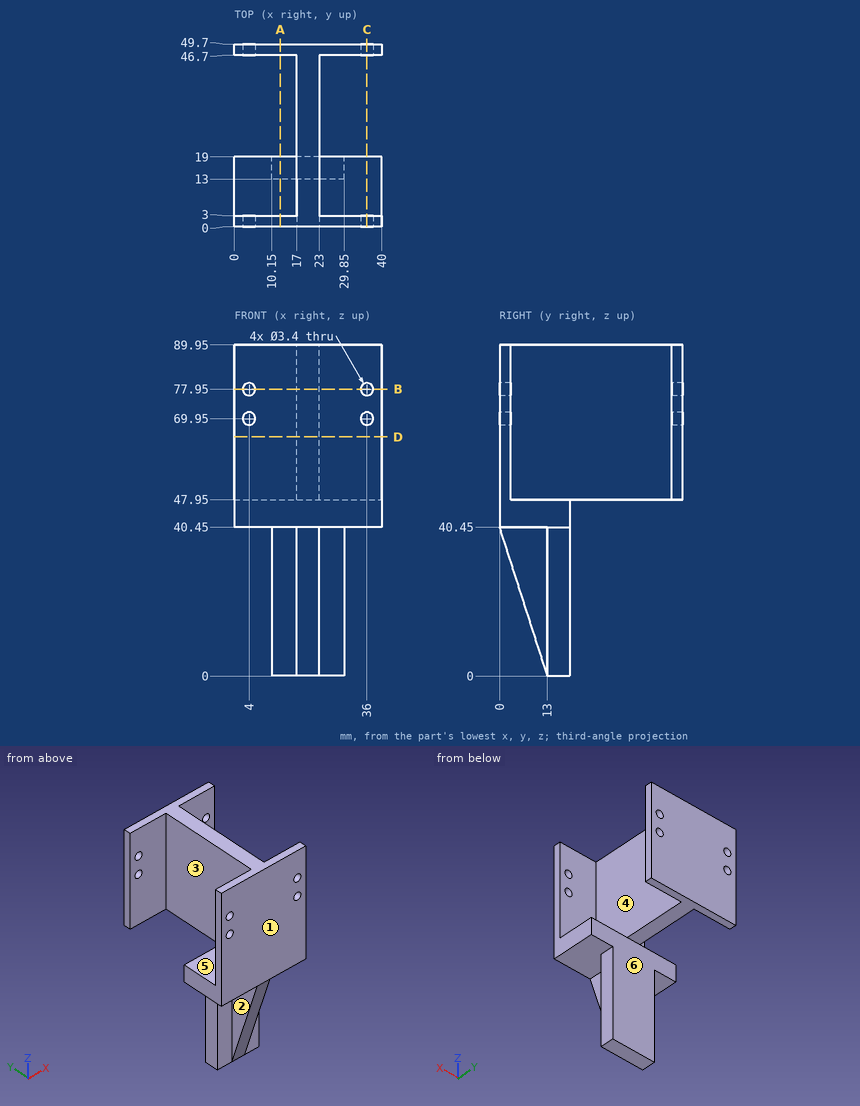
Could you check a few things on this drawing? It's one solid part, dimensions in mm from its lowest x, y, z. A direction names the side the tool comes from. Give positions to 0.01 mm unless a question says otherwise; leave off trailing zeros. Write each loop counter-clockwise with the first axis right and the second up, starting at its lowest first coordinate (ties: lowest second). Pieces come first, ordered by that corner, then holes.
(1) Imagine slicing it at B-B, the plane z = 77.95. Write out the boundary of the cut face in (x, y).
Output values:
outline: (0, 0) - (2.3, 0) - (2.3, 3) - (0, 3) - close; (0, 46.7) - (2.3, 46.7) - (2.3, 49.7) - (0, 49.7) - close; (5.7, 0) - (34.3, 0) - (34.3, 3) - (23, 3) - (23, 46.7) - (34.3, 46.7) - (34.3, 49.7) - (5.7, 49.7) - (5.7, 46.7) - (17, 46.7) - (17, 3) - (5.7, 3) - close; (37.7, 0) - (40, 0) - (40, 3) - (37.7, 3) - close; (37.7, 46.7) - (40, 46.7) - (40, 49.7) - (37.7, 49.7) - close
(2) Imagine slicing it at C-C, the plane x = 36. Write out the boundary of the cut face in (y, z), and give its area (3 significant figures).
Output values:
outline: (0, 40.45) - (19, 40.45) - (19, 47.95) - (3, 47.95) - (3, 68.25) - (0, 68.25) - close; (0, 71.65) - (3, 71.65) - (3, 76.25) - (0, 76.25) - close; (0, 79.65) - (3, 79.65) - (3, 89.95) - (0, 89.95) - close; (46.7, 47.95) - (49.7, 47.95) - (49.7, 68.25) - (46.7, 68.25) - close; (46.7, 71.65) - (49.7, 71.65) - (49.7, 76.25) - (46.7, 76.25) - close; (46.7, 79.65) - (49.7, 79.65) - (49.7, 89.95) - (46.7, 89.95) - close
area: 354 mm2
(3) Imagine slicing it at D-D, the plane z = 65. Write out the boundary of the cut face in (x, y), and give its area (3 significant figures).
Output values:
outline: (0, 0) - (40, 0) - (40, 3) - (23, 3) - (23, 46.7) - (40, 46.7) - (40, 49.7) - (0, 49.7) - (0, 46.7) - (17, 46.7) - (17, 3) - (0, 3) - close
area: 502 mm2
(4) Will these pins go through, and if not, where does the flat tip stop? pin 1 (4 mm diameter, centred on y = 7, z = 26.5, fed in from +X); pin 2 (12 mm diameter, centred on y = 23, z = 31.5, fed in from -X); pin 3 (1 mm diameter, centred on y = 9.5, z = 29, fed in from -X).
Output values:
pin 1: stops at x = 23
pin 2: stops at x = 10.15
pin 3: stops at x = 17
(5) On a 3-axis mill with a long thin cutter (end or side, diameter ignored), from which of +Z, -Z, +X, -X, +Y, -Y can I reach the whole of each face in a straight line? I mean the marked faces 4, 5 and 6. Say none if no direction works.
Output values:
face 4: +Z, +X
face 5: +Z, -X
face 6: -Z, +X, -X, +Y
(6) Thinking about a two-plate mould opening in Y: for the marked faces 1, 2 and 3, which applies, pulls with the +Y half, pulls with the -Y half, needs draft (parallel to the pull), parting line crosses it, or undercut?
Output values:
face 1: pulls with the -Y half
face 2: needs draft
face 3: undercut
(7) If I drill on L1, parallel to X at y = 47.7, z = 77.95; L2, parallel to X at y = 48, z = 69; L3, parallel to Y at x = 14.5, z = 79.5, over which ranges is the centre line in solid material (lowest first)?
Output values:
L1: x = 0 to 2.3, 5.7 to 34.3, 37.7 to 40
L2: x = 0 to 2.59, 5.41 to 34.59, 37.41 to 40
L3: y = 0 to 3, 46.7 to 49.7
(8) Imagine slicing it at A-A, the plane x = 12.5. Write out the boundary of the cut face in (y, z).
Output values:
outline: (0, 40.45) - (13, 40.45) - (13, 0) - (19, 0) - (19, 47.95) - (3, 47.95) - (3, 89.95) - (0, 89.95) - close; (46.7, 47.95) - (49.7, 47.95) - (49.7, 89.95) - (46.7, 89.95) - close
